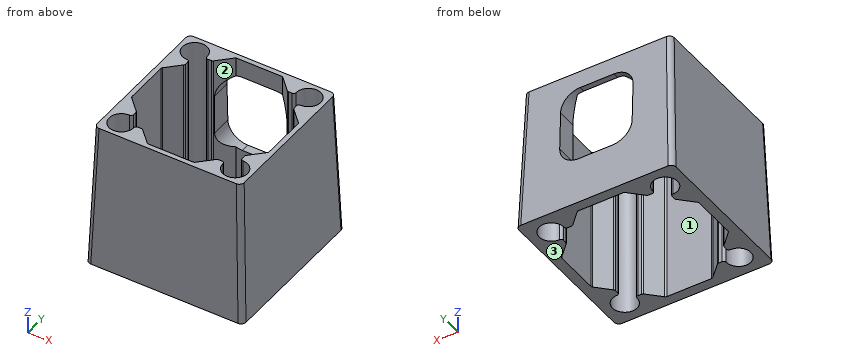
from build123d import *

# Parameters (mm, degrees)
SKETCH1_W           = 65
SKETCH1_H           = 65
BOSS_EXTRUDE1_DEPTH = 60
BOSS_EXTRUDE1_TAPER = 2
CUT_EXTRUDE1_REACH  = 77.581
SKETCH4_R           = 5.1
CUT_EXTRUDE2_REACH  = 77.581
SKETCH5_W           = 45
SKETCH5_H           = 45
CUT_EXTRUDE4_REACH  = 77.581
CUT_EXTRUDE5_REACH  = 95.495
SKETCH7_W           = 30
SKETCH7_H           = 32.536572658
FILLET1_R           = 2
FILLET3_R           = 1
FILLET5_R           = 8


with BuildPart() as part:
    # Sketch1 → Boss-Extrude1 (new body)
    with BuildSketch(Plane.XY):
        Rectangle(SKETCH1_W, SKETCH1_H)
    extrude(amount=BOSS_EXTRUDE1_DEPTH, taper=BOSS_EXTRUDE1_TAPER)

    # Sketch4 → Cut-Extrude1 (cut, up to next)
    with BuildSketch(Plane.XY.offset(60), mode=Mode.PRIVATE) as cut_extrude1_sk1:
        with Locations((-23.550191347, 23.550191347)):
            Circle(SKETCH4_R)
    cut_extrude1_tool1 = extrude(cut_extrude1_sk1.sketch, amount=-CUT_EXTRUDE1_REACH, mode=Mode.PRIVATE) & part.part
    # Sketch4 → Cut-Extrude1 (cut, up to next)
    with BuildSketch(Plane.XY.offset(60), mode=Mode.PRIVATE) as cut_extrude1_sk2:
        with Locations((23.550191347, 23.550191347)):
            Circle(SKETCH4_R)
    cut_extrude1_tool2 = extrude(cut_extrude1_sk2.sketch, amount=-CUT_EXTRUDE1_REACH, mode=Mode.PRIVATE) & part.part
    # Sketch4 → Cut-Extrude1 (cut, up to next)
    with BuildSketch(Plane.XY.offset(60), mode=Mode.PRIVATE) as cut_extrude1_sk3:
        with Locations((23.550191347, -23.550191347)):
            Circle(SKETCH4_R)
    cut_extrude1_tool3 = extrude(cut_extrude1_sk3.sketch, amount=-CUT_EXTRUDE1_REACH, mode=Mode.PRIVATE) & part.part
    # Sketch4 → Cut-Extrude1 (cut, up to next)
    with BuildSketch(Plane.XY.offset(60), mode=Mode.PRIVATE) as cut_extrude1_sk4:
        with Locations((-23.550191347, -23.550191347)):
            Circle(SKETCH4_R)
    cut_extrude1_tool4 = extrude(cut_extrude1_sk4.sketch, amount=-CUT_EXTRUDE1_REACH, mode=Mode.PRIVATE) & part.part
    add(cut_extrude1_tool1.solids().sort_by_distance((-23.550191, 23.550191, 60))[0], mode=Mode.SUBTRACT)
    add(cut_extrude1_tool2.solids().sort_by_distance((23.550191, 23.550191, 60))[0], mode=Mode.SUBTRACT)
    add(cut_extrude1_tool3.solids().sort_by_distance((23.550191, -23.550191, 60))[0], mode=Mode.SUBTRACT)
    add(cut_extrude1_tool4.solids().sort_by_distance((-23.550191, -23.550191, 60))[0], mode=Mode.SUBTRACT)

    # Sketch5 → Cut-Extrude2 (cut, up to next)
    with BuildSketch(Plane.XY.offset(60), mode=Mode.PRIVATE) as cut_extrude2_sk1:
        Rectangle(SKETCH5_W, SKETCH5_H)
    cut_extrude2_tool1 = extrude(cut_extrude2_sk1.sketch, amount=-CUT_EXTRUDE2_REACH, mode=Mode.PRIVATE) & part.part
    add(cut_extrude2_tool1.solids().sort_by_distance((0, 0, 60))[0], mode=Mode.SUBTRACT)

    # Sketch6 → Cut-Extrude4 (cut, up to next)
    with BuildSketch(Plane.XY.offset(60), mode=Mode.PRIVATE) as cut_extrude4_sk1:
        Polygon((-22.5, -15.559490181), (-22.5, 15.559490181), (-28.40475383, 9.65473635), (-28.40475383, -9.65473635), align=None)
    cut_extrude4_tool1 = extrude(cut_extrude4_sk1.sketch, amount=-CUT_EXTRUDE4_REACH, mode=Mode.PRIVATE) & part.part
    # Sketch6 → Cut-Extrude4 (cut, up to next)
    with BuildSketch(Plane.XY.offset(60), mode=Mode.PRIVATE) as cut_extrude4_sk2:
        Polygon((-15.559490181, 22.5), (15.559490181, 22.5), (9.65473635, 28.40475383), (-9.65473635, 28.40475383), align=None)
    cut_extrude4_tool2 = extrude(cut_extrude4_sk2.sketch, amount=-CUT_EXTRUDE4_REACH, mode=Mode.PRIVATE) & part.part
    # Sketch6 → Cut-Extrude4 (cut, up to next)
    with BuildSketch(Plane.XY.offset(60), mode=Mode.PRIVATE) as cut_extrude4_sk3:
        Polygon((22.5, 15.559490181), (22.5, -15.559490181), (28.40475383, -9.65473635), (28.40475383, 9.65473635), align=None)
    cut_extrude4_tool3 = extrude(cut_extrude4_sk3.sketch, amount=-CUT_EXTRUDE4_REACH, mode=Mode.PRIVATE) & part.part
    # Sketch6 → Cut-Extrude4 (cut, up to next)
    with BuildSketch(Plane.XY.offset(60), mode=Mode.PRIVATE) as cut_extrude4_sk4:
        Polygon((15.559490181, -22.5), (-15.559490181, -22.5), (-9.65473635, -28.40475383), (9.65473635, -28.40475383), align=None)
    cut_extrude4_tool4 = extrude(cut_extrude4_sk4.sketch, amount=-CUT_EXTRUDE4_REACH, mode=Mode.PRIVATE) & part.part
    add(cut_extrude4_tool1.solids().sort_by_distance((-25.221911, 0, 60))[0], mode=Mode.SUBTRACT)
    add(cut_extrude4_tool2.solids().sort_by_distance((0, 25.221911, 60))[0], mode=Mode.SUBTRACT)
    add(cut_extrude4_tool3.solids().sort_by_distance((25.221911, 0, 60))[0], mode=Mode.SUBTRACT)
    add(cut_extrude4_tool4.solids().sort_by_distance((0, -25.221911, 60))[0], mode=Mode.SUBTRACT)

    # Sketch7 → Cut-Extrude5 (cut, up to next)
    with BuildSketch(Plane(origin=(0, 32.460415817, 1.133542698), x_dir=(1, 0, 0), z_dir=(0, 0.9993908270190958, 0.034899496702501046)), mode=Mode.PRIVATE) as cut_extrude5_sk1:
        with Locations((0, -35.134052686)):
            Rectangle(SKETCH7_W, SKETCH7_H)
    cut_extrude5_tool1 = extrude(cut_extrude5_sk1.sketch, amount=-CUT_EXTRUDE5_REACH, mode=Mode.PRIVATE) & part.part
    add(cut_extrude5_tool1.solids().sort_by_distance((0, 31.234255, 36.246193))[0], mode=Mode.SUBTRACT)

    # Fillet1
    fillet1_edges = [part.edges().sort_by_distance(p)[0] for p in [
        (-31.452376453, 31.452376453, 30.000013228),
        (31.452376915, 31.452376915, 30),
        (31.452376453, -31.452376453, 30.000013228),
        (-31.452376915, -31.452376915, 30),
    ]]
    fillet(fillet1_edges, radius=FILLET1_R)

    # Fillet3
    fillet3_edges = [part.edges().sort_by_distance(p)[0] for p in [
        (-22.5, -15.559490181, 30),
        (-28.40475383, -9.65473635, 30),
        (-28.40475383, 9.65473635, 30),
        (-22.5, 15.559490181, 30),
        (-22.5, 18.559490181, 30),
        (-18.559490181, 22.5, 30),
        (18.559490181, 22.5, 30),
        (22.5, 18.559490181, 30),
        (22.5, -18.559490181, 30),
        (18.559490181, -22.5, 30),
        (-22.5, -18.559490181, 30),
        (-18.559490181, -22.5, 30),
        (15.559490181, -22.5, 30),
        (9.65473635, -28.40475383, 30),
        (-9.65473635, -28.40475383, 30),
        (-15.559490181, -22.5, 30),
        (-15.559490181, 22.5, 30),
        (15.559490181, 22.5, 30),
        (22.5, 15.559490181, 30),
        (28.40475383, 9.65473635, 30),
        (28.40475383, -9.65473635, 30),
        (22.5, -15.559490181, 30),
    ]]
    fillet(fillet3_edges, radius=FILLET3_R)

    # Fillet5
    fillet5_edges = [part.edges().sort_by_distance(p)[0] for p in [
        (15, 26.862995118, 52.371747478),
        (-15, 26.862995118, 52.371747478),
        (15, 27.430750123, 19.83516878),
        (-15, 27.430750123, 19.83516878),
    ]]
    fillet(fillet5_edges, radius=FILLET5_R)


solid = part.part
Geometry: final body of the model. Coordinates: model frame, mm. Face numbers are marked on the shaded views. Give positions to 0.01 mm unless a question says otherwise; leave off trailing zeros. Write each loop counter-clockwise with the first axis right and the second up, starting at its lowest first coordinate (ties: lowest second). Pieces come first, ordered by that corner, then holes. Notation, with made-up numbers: (-33.75, -1.75) -> (5.25, -1.75) arc R24 ccw to (5.25, 32.25) -> close; hole circle Ø1 at (-36, 63.5). An arc over 180 degrees is marked (long way). Answer as a JSON object with one key per item and string values.
1. Ray query, probe 1 along Y at (x, z) = (-26.5, 15); probe 2 along X at (y, z) = (-24.5, 55); probe 3 along Y at (x, z) = (-26, 14). Return the intervals inside material, ascending. Write a range as from..to.
Ans:
{"probe 1": "y = -31.98..-27.71, -19.39..-11.56, 11.56..19.39, 27.71..31.98", "probe 2": "x = -30.58..-28.56, -18.54..-13.56, 13.56..18.54, 28.56..30.58", "probe 3": "y = -32.01..-28.02, -19.08..-12.06, 12.06..19.08, 28.02..32.01"}
2. Mould query, pull axis X, two halves, no side actions, for the marked faces 1, 2 and 3. Classes: pulls with the +X half, pulls with the -X half, needs draft (parallel to the pull), parting line crosses it, or undercut.
Ans:
{"face 1": "undercut", "face 2": "undercut", "face 3": "needs draft"}
3. Cut plane A-A on x = -5. Output: boundary loops of the cut face in (y, z), and give its area (3 significant figures).
Ans:
{"outline": "(-32.5, 0) -> (-28.4, 0) -> (-28.4, 60) -> (-30.4, 60) -> close; (28.4, 0) -> (32.5, 0) -> (31.8, 19.99) -> (28.4, 19.87) -> close; (28.4, 52.43) -> (30.67, 52.5) -> (30.4, 60) -> (28.4, 60) -> close", "area": "274 mm^2"}
4. Cut plane C-C on x = -13.5. Output: boundary loops of the cut face in (y, z), and give its area (3 significant figures).
Ans:
{"outline": "(-32.5, 0) -> (-24.56, 0) -> (-24.56, 60) -> (-30.4, 60) -> close; (24.56, 0) -> (32.5, 0) -> (31.69, 23.32) -> (24.56, 23.07) -> close; (24.56, 48.95) -> (30.78, 49.17) -> (30.4, 60) -> (24.56, 60) -> close", "area": "654 mm^2"}
5. Contact query for flat-ended pins moving along their axis: pin 1 (1.2 mm diameter, centred on x = -17, z = 27.5, fed in from -Y); pin 2 (5 mm diameter, centred on x = -2.5, z = 23, fed in from +Y); pin 3 (9 mm diameter, centred on x = -23.55, y = 23.55, fed in from +Z); pin 4 (1.2 mm diameter, centred on x = -17, z = 40, fed in from +Y). Output: stop coordinate, or through.
Ans:
{"pin 1": "stops at y = -31.56", "pin 2": "stops at y = -28.4", "pin 3": "passes through", "pin 4": "stops at y = 31.12"}
6. Cut plane B-B on y = -0.5. Output: boundary loops of the cut face in (x, z), and give its area (3 significant figures).
Ans:
{"outline": "(-32.5, 0) -> (-28.4, 0) -> (-28.4, 60) -> (-30.4, 60) -> close; (28.4, 0) -> (32.5, 0) -> (30.4, 60) -> (28.4, 60) -> close", "area": "366 mm^2"}
7. Cut plane D-D on y = 21. Output: boundary loops of the cut face in (x, z).
Ans:
{"outline": "(-32.5, 0) -> (-27.97, 0) -> (-27.97, 60) -> (-30.4, 60) -> close; (27.97, 0) -> (32.5, 0) -> (30.4, 60) -> (27.97, 60) -> close"}
